Can you work these out from the model? Positions are in its coordinate system, mm. A direction names the side the tool comes from. Round coordinates to 2 decimals unless told otherwise and drop trailing zeros. Loops run counter-clockwise (first coordinate to the right, second up) from the corner with the lowest first, then second, coordinate; pieces in that order, holes last. Notation, with made-up numbers: (12.5, -27) -> (45.5, -27) arc R14 ccw to (45.5, -9) -> close; hole circle Ø1 at (-11, 49.5). An arc over 180 degrees is marked (long way). Write each question's results on one line, items separated by ' | '.
from build123d import *

# Parameters (mm, degrees)
EXTRUDE_1_DEPTH     = 10
SKETCH_3_R          = 4.5
SKETCH_3_R_2        = 2.5
EXTRUDE_2_DEPTH     = 120
SKETCH_4_R          = 1.5
CUT_EXTRUDE_1_DEPTH = 20
SKETCH_5_R          = 5
SKETCH_5_R_2        = 4.5
EXTRUDE_3_DEPTH     = 45
CUT_EXTRUDE_START   = -75
SKETCH_6_R          = 4.5
CUT_EXTRUDE_2_DEPTH = 75
CUT_EXTRUDE_START_2 = -18
SKETCH_7_R          = 5
CUT_EXTRUDE_3_DEPTH = 18


with BuildPart() as part:
    # 草图1 → 凸台-拉伸1 (new body)
    with BuildSketch(Plane.XY):
        Polygon((8, 0), (4, 6.92820323), (-4, 6.92820323), (-8, 0), (-4, -6.92820323), (4, -6.92820323), align=None)
    extrude(amount=EXTRUDE_1_DEPTH)

    # 草图3 → 凸台-拉伸2 (add)
    with BuildSketch(Plane(origin=(0, 0, 0), x_dir=(-1, 0, 0), z_dir=(0, 0, -1))):
        with Locations(Location((0, 0, 0), (0, 0, 180))):
            Circle(SKETCH_3_R)
        Circle(SKETCH_3_R_2, mode=Mode.SUBTRACT)
    extrude(amount=EXTRUDE_2_DEPTH)

    # 草图4 → 切除-拉伸1 (cut)
    with BuildSketch(Plane(origin=(0, 0, 0), x_dir=(1, 0, 0), z_dir=(0, 1, 0))):
        with Locations(Location((0, 110, 0), (0, 0, 270))):
            Circle(SKETCH_4_R)
    extrude(amount=-CUT_EXTRUDE_1_DEPTH, mode=Mode.SUBTRACT)

    # 草图5 → 凸台-拉伸3 (add)
    with BuildSketch(Plane(origin=(0, 0, 0), x_dir=(-1, 0, 0), z_dir=(0, 0, -1))):
        with Locations(Location((0, 0, 0), (0, 0, 180))):
            Circle(SKETCH_5_R)
        Circle(SKETCH_5_R_2, mode=Mode.SUBTRACT)
    extrude(amount=EXTRUDE_3_DEPTH)

    # 草图6 → 切除-拉伸2 (cut)
    with BuildSketch(Plane(origin=(0, 0, -120), x_dir=(-1, 0, 0), z_dir=(0, 0, -1)).offset(CUT_EXTRUDE_START)):
        Circle(SKETCH_6_R)
    extrude(amount=CUT_EXTRUDE_2_DEPTH, mode=Mode.SUBTRACT)

    # 草图7 → 切除-拉伸3 (cut)
    with BuildSketch(Plane(origin=(0, 0, -45), x_dir=(-1, 0, 0), z_dir=(0, 0, -1)).offset(CUT_EXTRUDE_START_2)):
        with Locations(Location((0, 0, 0), (0, 0, 180))):
            Circle(SKETCH_7_R)
    extrude(amount=CUT_EXTRUDE_3_DEPTH, mode=Mode.SUBTRACT)


solid = part.part
1. If we section it at C-C (z = -6): List the corners of the cut face in (x, y) for me, then the cut area to 3 significant figures.
Final values:
outline: circle Ø10 at (0, 0); hole circle Ø5 at (0, 0) | area: 58.9 mm2
2. If we section it at B-B (y = -2): List the corners of the cut face in (x, z) for me, then the cut area to 3 significant figures.
Final values:
outline: (-6.85, 0) -> (-4.58, 0) -> (-4.58, -27) -> (-1.5, -27) -> (-1.5, 0) -> (1.5, 0) -> (1.5, -27) -> (4.58, -27) -> (4.58, 0) -> (6.85, 0) -> (6.85, 10) -> (-6.85, 10) -> close | area: 303 mm2
3. If we section it at A-A (x = 0): List the corners of the cut face in (y, z) for me.
Final values:
outline: (-6.93, 0) -> (-5, 0) -> (-5, -27) -> (-2.5, -27) -> (-2.5, 0) -> (2.5, 0) -> (2.5, -27) -> (5, -27) -> (5, 0) -> (6.93, 0) -> (6.93, 10) -> (-6.93, 10) -> close
4. Will these pins go through, and if not, where does the flat tip stop? pin 1 (3 mm diameter, centred on x = 0.5, z = -12, fed in from -Y); pin 2 (6 mm diameter, centred on y = 5.5, z = -20.5, fed in from +X); pin 3 (4 mm diameter, centred on y = 5, z = 0.5, fed in from -X).
Final values:
pin 1: y = -5 | pin 2: x = 4.33 | pin 3: x = -6.27
5. On a 3-axis mill with a long thin cutter (end or side, diameter ignored), from which of +Z, -Z, +X, -X, +Y, -Y can I reach the whole of each face in a straight line? I mean faces 1 (the face through (-6.028, -3.416, 4.93)), 2 (the face through (0, 0, 0)). Say none if no direction works.
Final values:
face 1: +Z, -Z, -X, -Y | face 2: -Z
6. Please list where these lines run through material, in increasing order: line 1 (Y direction, x = 0, z = -11.75); line 2 (Z direction, x = 1.25, y = 0.5); line 3 (X direction, y = 1.75, z = 4.5). Write a range as from..to.
Final values:
line 1: -5..-2.5, 2.5..5 | line 2: 0..10 | line 3: -6.99..6.99
7. If we section it at D-D (y = 3.5): List the corners of the cut face in (x, z) for me.
Final values:
outline: (-5.98, 0) -> (-3.57, 0) -> (-3.57, -27) -> (3.57, -27) -> (3.57, 0) -> (5.98, 0) -> (5.98, 10) -> (-5.98, 10) -> close
8. We'd pull the mould along X, two halves only. Please class faces 3 (the face through (-5, 0, -13)), 4 (the face through (0, 0, 10)), 5 (the face through (0.54, -2.44, -13.31)): pulls with the +X half, pulls with the -X half, needs draft (parallel to the pull), parting line crosses it, or undercut.
Final values:
face 3: parting line crosses it | face 4: needs draft | face 5: undercut
